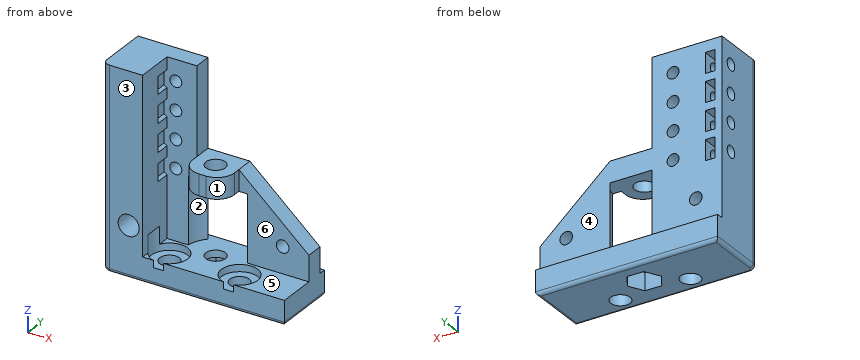
```python
from build123d import *

# Parameters (mm, degrees)
SKETCH_W        = 52
SKETCH_H        = 18
PAD_DEPTH       = 7
SKETCH001_W     = 52
SKETCH001_H     = 5
PAD001_DEPTH    = 50
SKETCH002_R     = 1.8
SKETCH002_W     = 12
SKETCH002_H     = 18
POCKET_DEPTH    = 5
SKETCH003_R     = 2.8
POCKET001_DEPTH = 7.001
SKETCH004_R     = 5.2
POCKET002_DEPTH = 2
SKETCH009_R     = 8.5
POCKET003_DEPTH = 19
POCKET004_DEPTH = 5
SKETCH006_W     = 12
SKETCH006_H     = 6
PAD002_DEPTH    = 7
SKETCH008_R     = 2.8
POCKET005_DEPTH = 32.001
SKETCH012_W     = 11.5
SKETCH012_H     = 50
PAD003_DEPTH    = 11
SKETCH013_R     = 3
POCKET006_DEPTH = 11
SKETCH014_R     = 5.2
POCKET007_DEPTH = 5
SKETCH015_R     = 1.7
POCKET008_DEPTH = 7
SKETCH016_R     = 1.7
SKETCH016_W     = 2.8
SKETCH016_H     = 5.8
POCKET009_DEPTH = 8
FILLET_R        = 5
FILLET001_R     = 2
FILLET002_R     = 1
POCKET010_DEPTH = 4


with BuildPart() as part:
    # Sketch → Pad (new body)
    with BuildSketch(Plane.XY):
        with Locations((0, -7)):
            Rectangle(SKETCH_W, SKETCH_H)
    extrude(amount=PAD_DEPTH)

    # Sketch001 → Pad001 (new body)
    with BuildSketch(Plane.XY.offset(7)):
        with Locations((0, -2.5)):
            Rectangle(SKETCH001_W, SKETCH001_H)
    extrude(amount=PAD001_DEPTH)

    # Sketch002 → Pocket (cut)
    with BuildSketch(Plane.XZ.offset(5)):
        with Locations((-18.5, 14.5)):
            Circle(SKETCH002_R)
        with Locations((18.5, 14.5)):
            Circle(SKETCH002_R)
        with Locations((0, 16)):
            Rectangle(SKETCH002_W, SKETCH002_H)
        Polygon((6, 32), (26.350149, 14), (26.350149, 32), (26.350149, 59.239628), (-6, 59.239628), (-6, 32), align=None)
    extrude(amount=-POCKET_DEPTH, mode=Mode.SUBTRACT)

    # Sketch003 → Pocket001 (cut, through all)
    with BuildSketch(Plane.XY.offset(7)):
        with Locations((0, -6)):
            Circle(SKETCH003_R)
        with Locations((10, -11)):
            Circle(SKETCH003_R)
        with Locations((-10, -11)):
            Circle(SKETCH003_R)
    extrude(amount=-POCKET001_DEPTH, mode=Mode.SUBTRACT)

    # Sketch004 → Pocket002 (cut)
    with BuildSketch(Plane.XY.offset(7)):
        with Locations((-10, -11)):
            Circle(SKETCH004_R)
        with Locations((10, -11)):
            Circle(SKETCH004_R)
    extrude(amount=-POCKET002_DEPTH, mode=Mode.SUBTRACT)

    # Sketch009 → Pocket003 (cut)
    with BuildSketch(Plane.XY.offset(7)):
        with Locations((0, -6)):
            Circle(SKETCH009_R)
    extrude(amount=POCKET003_DEPTH, mode=Mode.SUBTRACT)

    # Sketch005 → Pocket004 (cut)
    with BuildSketch(Plane(origin=(0, 0, 0), x_dir=(1, 0, 0), z_dir=(0, 0, -1))):
        Polygon((4.791368, 5.921741), (2.463458, 10.110317), (-2.32791, 10.188576), (-4.791368, 6.078259), (-2.463458, 1.889683), (2.32791, 1.811424), align=None)
    extrude(amount=-POCKET004_DEPTH, mode=Mode.SUBTRACT)

    # Sketch006 → Pad002 (new body)
    with BuildSketch(Plane.XZ.offset(5)):
        with Locations((0, 29)):
            Rectangle(SKETCH006_W, SKETCH006_H)
    extrude(amount=PAD002_DEPTH)

    # Sketch008 → Pocket005 (cut, through all)
    with BuildSketch(Plane.XY.offset(32)):
        with Locations((0, -6)):
            Circle(SKETCH008_R)
    extrude(amount=-POCKET005_DEPTH, mode=Mode.SUBTRACT)

    # Sketch012 → Pad003 (new body)
    with BuildSketch(Plane.XZ.offset(5)):
        with Locations((-20.25, 32)):
            Rectangle(SKETCH012_W, SKETCH012_H)
    extrude(amount=PAD003_DEPTH)

    # Sketch013 → Pocket006 (cut)
    with BuildSketch(Plane.XZ.offset(16)):
        with Locations((-18.5, 14.5)):
            Circle(SKETCH013_R)
    extrude(amount=-POCKET006_DEPTH, mode=Mode.SUBTRACT)

    # Sketch014 → Pocket007 (cut)
    with BuildSketch(Plane.XY.offset(7)):
        with Locations((-10, -11)):
            Circle(SKETCH014_R)
    extrude(amount=POCKET007_DEPTH, mode=Mode.SUBTRACT)

    # Sketch015 → Pocket008 (cut)
    with BuildSketch(Plane(origin=(-26, 0, 0), x_dir=(0, -1, 0), z_dir=(-1, 0, 0))):
        with Locations((4, 51)):
            Circle(SKETCH015_R)
        with Locations((4, 43)):
            Circle(SKETCH015_R)
        with Locations((4, 35)):
            Circle(SKETCH015_R)
        with Locations((4, 27)):
            Circle(SKETCH015_R)
    extrude(amount=-POCKET008_DEPTH, mode=Mode.SUBTRACT)

    # Sketch016 → Pocket009 (cut)
    with BuildSketch(Plane(origin=(0, 0, 0), x_dir=(-1, 0, 0), z_dir=(0, 1, 0))):
        with Locations((12, 51)):
            Circle(SKETCH016_R)
        with Locations((12, 43)):
            Circle(SKETCH016_R)
        with Locations((12, 35)):
            Circle(SKETCH016_R)
        with Locations((12, 27)):
            Circle(SKETCH016_R)
        with Locations((22.6, 50.981492)):
            Rectangle(SKETCH016_W, SKETCH016_H)
        with Locations((22.6, 42.981492)):
            Rectangle(SKETCH016_W, SKETCH016_H)
        with Locations((22.6, 34.981492)):
            Rectangle(SKETCH016_W, SKETCH016_H)
        with Locations((22.6, 26.981492)):
            Rectangle(SKETCH016_W, SKETCH016_H)
    extrude(amount=-POCKET009_DEPTH, mode=Mode.SUBTRACT)

    # Fillet
    fillet_edges = [part.edges().sort_by_distance(p)[0] for p in [
        (-6, -12, 29),
        (6, -12, 29),
    ]]
    fillet(fillet_edges, radius=FILLET_R)

    # Fillet001
    fillet001_edges = [part.edges().sort_by_distance(p)[0] for p in [
        (-26, -16, 28.5),
    ]]
    fillet(fillet001_edges, radius=FILLET001_R)

    # Fillet002
    fillet002_edges = [part.edges().sort_by_distance(p)[0] for p in [
        (26, -7, 0),
        (1, -16, 0),
        (0, 2, 0),
        (-26, -6, 0),
    ]]
    fillet(fillet002_edges, radius=FILLET002_R)

    # Sketch017 → Pocket010 (cut)
    with BuildSketch(Plane.XZ.offset(5)):
        Polygon((-8.6, 49.037009), (-8.6, 52.962991), (-12, 54.925982), (-15.4, 52.962991), (-15.4, 49.037009), (-12, 47.074018), align=None)
        Polygon((-8.6, 41.037009), (-8.6, 44.962991), (-12, 46.925982), (-15.4, 44.962991), (-15.4, 41.037009), (-12, 39.074018), align=None)
        Polygon((-8.6, 33.037009), (-8.6, 36.962991), (-12, 38.925982), (-15.4, 36.962991), (-15.4, 33.037009), (-12, 31.074018), align=None)
        Polygon((-8.6, 25.037009), (-8.6, 28.962991), (-12, 30.925982), (-15.4, 28.962991), (-15.4, 25.037009), (-12, 23.074018), align=None)
    extrude(amount=POCKET010_DEPTH, mode=Mode.SUBTRACT)


solid = part.part
```
Geometry check sheet. Reference: the model listing, model coordinates, mm. Face numbers are marked on the shaded views. A direction names the side the tool comes from. Coordinates: 2 decimals unless noted, no trailing zeros. Loops run counter-clockwise (first coordinate to the right, second up) from the corner with the lowest first, then second, coordinate; pieces in that order, holes last.
Item 1: Release check for a two-part mould opening along X. For the marked faces 1, 2 and 3 record: released by +X, released by -X, zero draft, split by the parting line, or undercut.
Item 2: Sectioned sample at B-B, the plane x = 19. Record the boundary of the cut face in (y, z).
Item 3: Access from +Z, -Z, +X, -X, +Y, -Y to the whole of each face (thin tool, end or side, straight path). Record for the marked faces 4, 5 and 6.
Item 4: Sectioned sample at C-C, the plane x = 0. Record the boundary of the cut face in (y, z), then the cut area to 3 significant figures.
Item 5: Sectioned sample at A-A, the plane z = 43. Record the boundary of the cut face in (x, y), then the cut area to 3 significant figures.
Item 6: Sectioned sample at D-D, the plane y = -4. Count the separate pieces of the cut face and the enclosed holes in it, then the cut area to 3 significant figures.
Item 7: Thickness scan on line 1 (X direction, y = -11, z = 6.05); line 2 (Z direction, x = -19.8, y = -4); line 3 (Z direction, x = -13, y = -2.5). Record the ranges inside material, lowest first.
Item 8: Go/stop test with flat-tipped pins: pin 1 Ø8 at (y, z) = (-7.5, 43) entering from +X; pin 2 Ø1 at (y, z) = (-4.5, 34.5) entering from -X; pin 3 Ø4 at (x, z) = (-10, 15) entering from -Y. Record where each tip stops, or that it passes through.
Check result:
1. face 1: released by +X
1. face 2: undercut
1. face 3: zero draft
2. outline: (-16, 1) arc R1 ccw to (-15, 0) - (1, 0) arc R1 ccw to (2, 1) - (2, 7) - (0, 7) - (0, 12.77) - (-5, 12.77) - (-5, 7) - (-16, 7) - close; (-5, 16.23) - (0, 16.23) - (0, 20.5) - (-5, 20.5) - close
3. face 4: +Z, +X, -X, +Y
3. face 5: none
3. face 6: +Z, +X, -Y
4. outline: (-16, 1) arc R1 ccw to (-15, 0) - (-10.15, 0) - (-10.15, 5) - (-8.8, 5) - (-8.8, 7) - (-16, 7) - close; (-12, 26) - (-8.8, 26) - (-8.8, 32) - (-12, 32) - close; (-3.2, 5) - (-1.85, 5) - (-1.85, 0) - (1, 0) arc R1 ccw to (2, 1) - (2, 7) - (-3.2, 7) - close; (-3.2, 26) - (0, 26) - (0, 32) - (-3.2, 32) - close
4. area: 111 mm2
5. outline: (-26, -14) arc R2 ccw to (-24, -16) - (-14.5, -16) - (-14.5, -9) - (-15.4, -9) - (-15.4, -5) - (-13.7, -5) - (-13.7, 0) - (-21.2, 0) - (-21.2, -2.3) - (-19, -2.3) - (-19, -5.7) - (-21.2, -5.7) - (-21.2, -8) - (-24, -8) - (-24, -5.7) - (-26, -5.7) - close; (-26, -2.3) - (-24, -2.3) - (-24, 0) - (-26, 0) - close; (-10.3, -5) - (-6, -5) - (-6, 0) - (-10.3, 0) - close
5. area: 168 mm2
6. separate pieces: 2
6. enclosed holes: 6
6. area: 1,430 mm2
7. line 1: x = -26 to -15.2, -4.8 to 4.8, 15.2 to 26
7. line 2: z = 0 to 13.26, 15.74 to 25.3, 28.7 to 33.3, 36.7 to 41.3, 44.7 to 49.3, 52.7 to 57
7. line 3: z = 0 to 25.63, 28.37 to 33.63, 36.37 to 41.63, 44.37 to 49.63, 52.37 to 57
8. pin 1: stops at x = -6
8. pin 2: stops at x = -19
8. pin 3: stops at y = -5
